```python
from build123d import *

# Parameters (mm, degrees)
SKETCH1_R           = 90
SKETCH1_R_2         = 44.5
BOSS_EXTRUDE1_DEPTH = 80
FILLET1_R           = 15
FILLET2_R           = 10


with BuildPart() as part:
    # Sketch1 → Boss-Extrude1 (new body)
    with BuildSketch(Plane(origin=(0, 0, 0), x_dir=(1, 0, 0), z_dir=(0, 1, 0))):
        Circle(SKETCH1_R)
        Circle(SKETCH1_R_2, mode=Mode.SUBTRACT)
    extrude(amount=BOSS_EXTRUDE1_DEPTH)

    # Sketch2 → Cut-Revolve1 (revolve, cut)
    with BuildSketch(Plane.XY):
        Polygon((61.5, 0), (49.5, 11.75), (44.5, 11.75), (44.5, 0), align=None)
    cut_revolve1 = revolve(axis=Axis((0, 0, 0), (0, 1, 0)), mode=Mode.SUBTRACT)

    # Mirror1: Cut-Revolve1 across plane
    add(cut_revolve1.mirror(Plane(origin=(0, 40, 0), x_dir=(0, 0, 1), z_dir=(0, -1, 0))), mode=Mode.SUBTRACT)

    # Fillet1
    fillet1_edges = [part.edges().sort_by_distance(p)[0] for p in [
        (-61.5, 0, 0),
        (-61.5, 80, 0),
    ]]
    fillet(fillet1_edges, radius=FILLET1_R)

    # Fillet2
    fillet2_edges = [part.edges().sort_by_distance(p)[0] for p in [
        (-90, 0, 0),
        (-90, 80, 0),
    ]]
    fillet(fillet2_edges, radius=FILLET2_R)


solid = part.part
```
CAD build for the part. Positions are in the model's coordinates, mm. A direction names the side the tool comes from. Round coordinates to 2 decimals unless told otherwise and drop trailing zeros. Write each loop counter-clockwise with the first axis right and the second up, starting at its lowest first coordinate (ties: lowest second). Pieces come first, ordered by that corner, then holes. Notation, with made-up numbers: (56, 57) -> (101, 57) arc R19 cw to (101, 83) -> close; hole circle Ø2 at (56.5, -34.75). An arc over 180 degrees is marked (long way). Answer in a Markdown table with one row per item. Add a question column.
Item 1: Saw through at A-A, the plane x = 0. Write the cut outline in (y, z).
Item 2: Saw through at C-C, the plane y = 46. Write the cut outline in (x, z), then the cut area to 3 significant figures.
Item 3: Which spindle directions (+Z, -Z, +X, -X, +Y, -Y) get a long thin tool onto all of the face, cutting with end or side? Do faces 4 (the face through (-32.798, 39.604, -30.075)), 5 (the face through (-41, 11.75, -19)), 6 (the face through (-41, 68.25, -19)). Say none if no direction does.
Item 4: Drill centre lines: line 1 (Z direction, x = 0, y = 33); line 2 (Z direction, x = -37, y = 18). Where is each one in solid material? Low to high. Write a range as from..to.
Item 5: Mould opens along Z. For faces 1 (the face through (41.53, 39.58, 79.845)), 2 (the face through (-18, 0, -66)), 3 (the face through (-39.575, 68.613, 30.345)) say: pulls with the +Z half, pulls with the -Z half, needs draft (parallel to the pull), parting line crosses it, or undercut.
Item 6: Saw through at B-B, the plane z = 0. Write the cut outline in (x, y), then the cut area to 3 significant figures.
Item 7: Drop flat-ended pins along their axis: pin 1 Ø12 at (x, y) = (62, 54.5) entering from -Z; pin 2 Ø2 at (y, z) = (58, 24.5) entering from +X; pin 3 Ø3 at (x, y) = (-38, 45) entering from +Z. Give the stop position or say it passes through.
Findings below:
| question | item | result |
|---|---|---|
| 1 | outline | (0, -80) arc R10 ccw to (10, -90) -> (70, -90) arc R10 ccw to (80, -80) -> (80, -67.62) arc R15 ccw to (75.72, -57.13) -> (68.25, -49.5) -> (68.25, -44.5) -> (11.75, -44.5) -> (11.75, -49.5) -> (4.28, -57.13) arc R15 ccw to (0, -67.62) -> close; (0, 67.62) arc R15 ccw to (4.28, 57.13) -> (11.75, 49.5) -> (11.75, 44.5) -> (68.25, 44.5) -> (68.25, 49.5) -> (75.72, 57.13) arc R15 ccw to (80, 67.62) -> (80, 80) arc R10 ccw to (70, 90) -> (10, 90) arc R10 ccw to (0, 80) -> close |
| 2 | outline | circle Ø180 at (0, 0); hole circle Ø89 at (0, 0) |
| 2 | area | 19,200 mm^2 |
| 3 | face 4 | +Y, -Y |
| 3 | face 5 | -Y |
| 3 | face 6 | +Y |
| 4 | line 1 | z = -90..-44.5, 44.5..90 |
| 4 | line 2 | z = -82.04..-24.72, 24.72..82.04 |
| 5 | face 1 | parting line crosses it |
| 5 | face 2 | needs draft |
| 5 | face 3 | undercut |
| 6 | outline | (-90, 10) arc R10 ccw to (-80, 0) -> (-67.62, 0) arc R15 ccw to (-57.13, 4.28) -> (-49.5, 11.75) -> (-44.5, 11.75) -> (-44.5, 68.25) -> (-49.5, 68.25) -> (-57.13, 75.72) arc R15 ccw to (-67.62, 80) -> (-80, 80) arc R10 ccw to (-90, 70) -> close; (44.5, 11.75) -> (49.5, 11.75) -> (57.13, 4.28) arc R15 ccw to (67.62, 0) -> (80, 0) arc R10 ccw to (90, 10) -> (90, 70) arc R10 ccw to (80, 80) -> (67.62, 80) arc R15 ccw to (57.13, 75.72) -> (49.5, 68.25) -> (44.5, 68.25) -> close |
| 6 | area | 6,660 mm^2 |
| 7 | pin 1 | stops at z = -70.46 |
| 7 | pin 2 | stops at x = 86.88 |
| 7 | pin 3 | stops at z = 82.27 |
